```python
from build123d import *

# Parameters (mm, degrees)
SKETCH1_W           = 3
SKETCH1_H           = 16
BOSS_EXTRUDE1_DEPTH = 3
SKETCH2_W           = 40
SKETCH2_H           = 1.6
BOSS_EXTRUDE2_DEPTH = 3
SKETCH3_R           = 15.651050508
SKETCH3_R_2         = 13.636404617
SKETCH3_R_3         = 9.625367155
SKETCH3_R_4         = 8.055659383
SKETCH3_R_5         = 8.6792975
SKETCH3_R_6         = 6.974005881
SKETCH3_R_7         = 2.446418815
SKETCH3_R_8         = 3.779523595
SKETCH3_R_9         = 2.94345793
CUT_EXTRUDE1_DEPTH  = 10


with BuildPart() as part:
    # Sketch1 → Boss-Extrude1 (new body)
    with BuildSketch(Plane(origin=(0, 0, 0), x_dir=(0, 0, -1), z_dir=(1, 0, 0))):
        Polygon((30, -40), (180, -8), (180, -3), (146.666666667, -3), (146.666666667, 0), (106.666666667, 0), (106.666666667, -3), (73.333333333, -3), (73.333333333, 0), (33.333333333, 0), (33.333333333, -3), (0, -3), (0, 0), (-4, 0), (-4, -40), (0, -40), align=None)
        with Locations((1.5, -20)):
            Rectangle(SKETCH1_W, SKETCH1_H, mode=Mode.SUBTRACT)
    extrude(amount=BOSS_EXTRUDE1_DEPTH)

    # Sketch2 → Boss-Extrude2 (add)
    with BuildSketch(Plane(origin=(3, 0, 0), x_dir=(0, 0, -1), z_dir=(1, 0, 0))):
        with Locations((126.666666667, 0.8)):
            Rectangle(SKETCH2_W, SKETCH2_H)
    extrude(amount=-BOSS_EXTRUDE2_DEPTH)

    # Sketch3 → Cut-Extrude1 (cut)
    with BuildSketch(Plane(origin=(3, 0, 0), x_dir=(0, 0, -1), z_dir=(1, 0, 0))):
        with Locations((22.104563443, -20.956095071)):
            Circle(SKETCH3_R)
        with Locations((54.328943076, -16.752253971)):
            Circle(SKETCH3_R_2)
        with Locations((82.483117774, -15.673188709)):
            Circle(SKETCH3_R_3)
        with Locations((103.057816826, -13.060067591)):
            Circle(SKETCH3_R_4)
        with Locations((120.792027676, -9.128318411)):
            Circle(SKETCH3_R_5)
        with Locations((138.707850434, -7.192260379)):
            Circle(SKETCH3_R_6)
        with Locations((168.340077715, -6.548539538)):
            Circle(SKETCH3_R_7)
        with Locations((152.117415019, -8.502294699)):
            Circle(SKETCH3_R_8)
        with Locations((160.801244487, -7.420684272)):
            Circle(SKETCH3_R_9)
    extrude(amount=-CUT_EXTRUDE1_DEPTH, mode=Mode.SUBTRACT)


solid = part.part
```
Design review of the part built by this model. Coordinates are the model's own, in mm. A direction names the side the tool comes from. Coordinates: 2 decimals unless noted, no trailing zeros. Write each loop counter-clockwise with the first axis right and the second up, starting at its lowest first coordinate (ties: lowest second). Pieces come first, ordered by that corner, then holes. Notation, with made-up numbers: M 61,-34.5 L 76,-34.5 A21 ccw 76,-28.5 Z; hole C -5,57 d4. An arc over 180 degrees is marked long. Answer as a JSON object with one key per item and string values.
Item 1: Add section A-A, the plane z = -8.5. Give the boundary of the cut face in (x, y), and give its area (3 significant figures).
Outcome:
{"outline": "M 0,-40 L 3,-40 L 3,-28.69 L 0,-28.69 Z; M 0,-13.22 L 3,-13.22 L 3,-3 L 0,-3 Z", "area": "64.6 mm²"}
Item 2: Add section B-B, the plane x = 1.7. State how many separate pieces and enclosed holes the cut face has, and give its area (3 significant figures).
Outcome:
{"separate pieces": "1", "enclosed holes": "10", "area": "2,350 mm²"}
Item 3: Draft analysis for pull direction Y (two halves, no side actions). For faces 1 (the flat face through (1, 0, 2)), 2 (the cylindrical face through (1.52, -6.89, -131.74)), 3 (the flat face through (1.479, -24.224, -103.95)), state which applies: pulls with the +Y half, pulls with the -Y half, needs draft (parallel to the pull), parting line crosses it, or undercut.
Outcome:
{"face 1": "pulls with the +Y half", "face 2": "undercut", "face 3": "pulls with the -Y half"}
Item 4: Wall thickness on probe 1 along Y at (x, z) = (2.1, -5); probe 2 along Z at (x, y) = (1.2, -1.5); probe 3 along Y at (x, z) = (0.25, -151): over which ranges is each line inside the solid? List them lowest first.
Outcome:
{"probe 1": "-40 to -3", "probe 2": "-146.67 to -142.74, -134.68 to -124.93, -116.65 to -106.67, -73.33 to -33.33, 0 to 4", "probe 3": "-14.19 to -12.11, -4.89 to -3"}
Item 5: Add section C-C, the plane z = -57.5. Give the boundary of the cut face in (x, y).
Outcome:
{"outline": "M 0,-34.13 L 3,-34.13 L 3,-30.01 L 0,-30.01 Z; M 0,-3.49 L 3,-3.49 L 3,0 L 0,0 Z"}
Item 6: Insertion check: pin 1 Ø4 at (y, z) = (-6.55, -168.34) entering from +X; pin 2 Ø1 at (x, z) = (2.5, -150.5) entering from -Y; pin 3 Ø1.5 at (x, y) = (1, -2) entering from -Z; pin 4 Ø0.9 at (x, z) = (1.5, -52) entering from +Y. Each pin has a flat end and moves straight along its axis. Give the tip position at first contact, or say it passes through.
Outcome:
{"pin 1": "through", "pin 2": "y = -14.4", "pin 3": "z = -146.67", "pin 4": "y = 0"}
Item 7: Machinability: for faces 4 (the flat face through (2, -1, -106.667)), 5 (the flat face through (1, -3, -164)), 6 (the flat face through (1, -20, 0)), 7 (the flat face through (1, 0, -54)), which of the approach directions +Z, -Z, +X, -X, +Y, -Y give a long, thin tool a straight path to every point of the face, cutting with its end or side? Answer none if there is none.
Outcome:
{"face 4": "+X, -X, +Y", "face 5": "-Z, +X, -X, +Y", "face 6": "+X, -X", "face 7": "+Z, +X, -X, +Y"}
